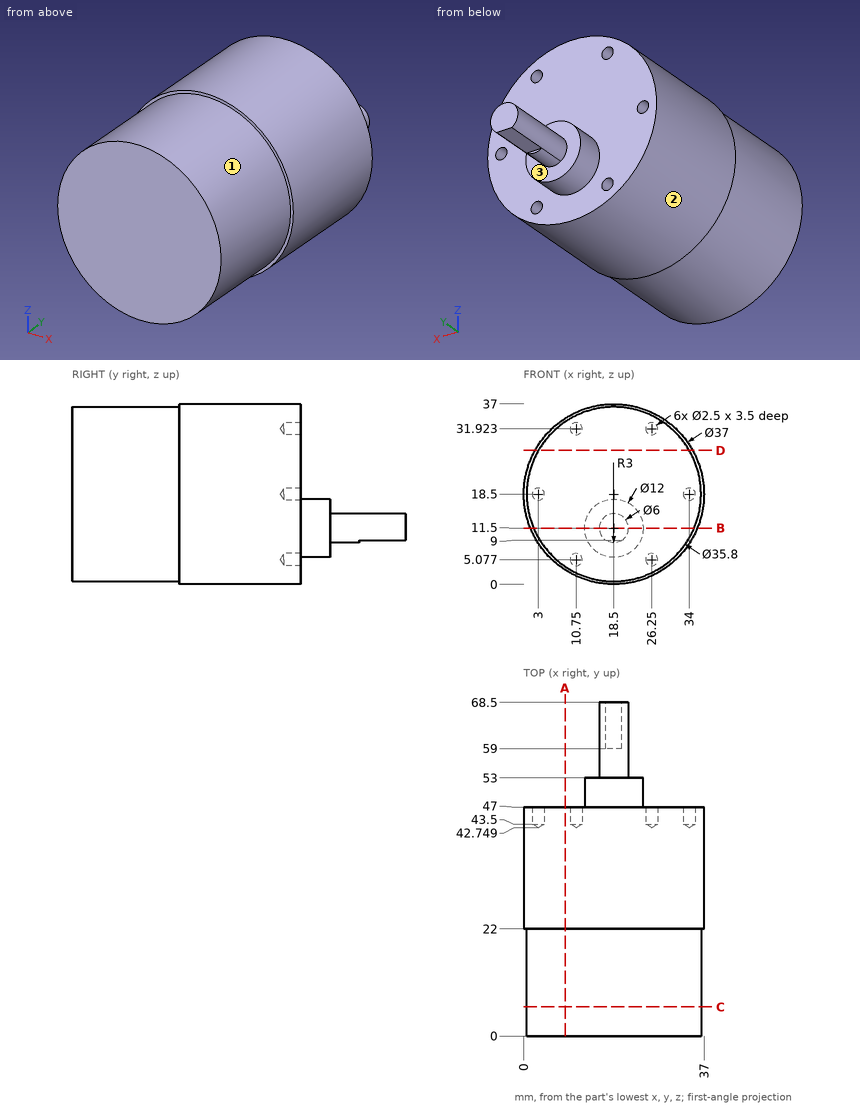
Geometry check sheet. Reference: drawing and pictorial views, mm from the part's lowest x, y, z. A direction names the side the tool comes from. Give positions to 0.01 mm unless a question says otherwise; leave off trailing zeros. Loops run counter-clockwise (first coordinate to the right, second up) from the corner with the lowest first, then second, coordinate; pieces in that order, holes last. Notation, with made-up numbers: (77, 69.25) - (106, 69.25) arc R22 ccw to (106, 94.25) - close; hole circle Ø9 at (-20.5, -30). An arc over 180 degrees is marked (long way). One line per question, with ' | ' between items. Start each with the question number.
1. Gauge pin test, flat ends, axial feed: pin 1 Ø6 at (x, z) = (13, 31.5) entering from +Y; pin 2 Ø1.5 at (x, y) = (26.5, 36) entering from -Z; pin 3 Ø3 at (x, y) = (15, 7.5) entering from -Z. Record the tip position at first contact, or that the pin passes through.
2. Cross-section at A-A, the plane x = 8.5. Enter the section's corners in (y, z) (1 decimal), plus the area to 3 significant figures.
3. Cross-section at B-B, the plane z = 11.5. Enter the section's corners in (x, y) (1 decimal), plus the area to 3 significant figures.
4. Set-up check for the marked faces 1, 2 and 3: record each of +Z, -Z, +X, -X, +Y, -Y from which the full face is reachable in a straight line by a thin tool's end or side.
5. Material ranges on line 1 along X through (y, z) = (45.95, 18.5); line 2 along Z through (x, y) = (26, 45); line 3 along Z through (x, y) = (26.25, 45.3), recorded low to high. Write a range as [from, to].
6. Cross-section at C-C, the plane y = 6. Enter the section's corners in (x, z).
7. Cross-section at D-D, the plane z = 27.5. Enter the section's corners in (x, y).
Check result:
1) pin 1: stops at y = 47 | pin 2: stops at z = 1.48 | pin 3: stops at z = 0.71
2) outline: (0, 3.7) - (22, 3.7) - (22, 2.9) - (47, 2.9) - (47, 34.1) - (22, 34.1) - (22, 33.3) - (0, 33.3) - close | area: 1,430 mm2
3) outline: (1.4, 22) - (2, 22) - (2, 0) - (35, 0) - (35, 22) - (35.6, 22) - (35.6, 47) - (24.5, 47) - (24.5, 53) - (21.5, 53) - (21.5, 68.5) - (15.5, 68.5) - (15.5, 53) - (12.5, 53) - (12.5, 47) - (1.4, 47) - close | area: 1,750 mm2
4) face 1: -Y | face 2: +Y, -Y | face 3: +Y
5) line 1: x = [0, 1.75], [4.25, 32.75], [35.25, 37] | line 2: z = [1.59, 3.85], [6.3, 30.7], [33.15, 35.41] | line 3: z = [1.7, 3.83], [6.33, 30.67], [33.17, 35.3]
6) outline: circle Ø35.8 at (18.5, 18.5)
7) outline: (2.34, 22) - (3.03, 22) - (3.03, 0) - (33.97, 0) - (33.97, 22) - (34.66, 22) - (34.66, 47) - (2.34, 47) - close
